Here's how the part is built. I have some questions about the finished solid (model axes, mm). Face numbers are marked on the shaded views. A direction names the side the tool comes from. Coordinates: 2 decimals unless noted, no trailing zeros.
```python
from build123d import *

# Parameters (mm, degrees)
SKETCH1_W                        = 15
SKETCH1_H                        = 6
MAIN_BODY_EXT_DEPTH              = 8.3
EMISSION_PATH_EXT_DEPTH          = 9
SKETCH3_R                        = 1.25
EMISSION_AND_GRIN_CUT_DEPTH      = 20.092931
SKETCH4_R                        = 1
DRUM_LENS_CUT_DEPTH              = 13
SKETCH41_R                       = 1
ADDTL_LIGHT_SOURCE_DEPTH         = 5
SKETCH5_W                        = 15
SKETCH5_H                        = 7.3
FILTERSET_CUT1_DEPTH             = 1
FILTERSET_CUT2_DEPTH             = 4
SKETCH10_R                       = 2.5
EMISSION_LENS_CUT_DEPTH          = 8.5
SKETCH15_R                       = 0.795
MAGNETS_CUT_DEPTH                = 0.9
SCREW_HOLES_CUT_DEPTH            = 20.507434
SCREW_HOLES_CUT_DEPTH_BACK       = 3
SKETCH18_R                       = 0.375
EXTERNAL_FILLET_1_R              = 1.5
CUT_EXTRUDE8_DEPTH               = 14.011149
CUT_EXTRUDE8_DEPTH_BACK          = 4
SKETCH28_R                       = 1.5
CUT_EXTRUDE9_DEPTH               = 3
CUT_EXTRUDE_ORIGINAL_LIGHT_DEPTH = 0.7
CUT_EXTRUDE_ADDTL_LIGHT_DEPTH    = 0.7
SKETCH29_R                       = 0.375
CUT_EXTRUDE11_DEPTH              = 2.5
SKETCH32_W                       = 2
SKETCH32_H                       = 2.36
CUT_EXTRUDE14_DEPTH              = 0.7
SKETCH45_W                       = 2.36
SKETCH45_H                       = 2
CUT_EXTRUDE19_DEPTH              = 0.7
CUT_EXTRUDE16_DEPTH              = 9
CUT_EXTRUDE17_REACH              = 13.945
SKETCH37_R                       = 2
BOSS_EXTRUDE2_DEPTH              = 1
SKETCH51_R                       = 0.356741
ADD_L_SCREW_HOLE_DEPTH           = 2


with BuildPart() as part:
    # Sketch1 → Main Body Ext (new body)
    with BuildSketch(Plane(origin=(0, 0, 0), x_dir=(1, 0, 0), z_dir=(0, 1, 0))):
        Rectangle(SKETCH1_W, SKETCH1_H)
    extrude(amount=MAIN_BODY_EXT_DEPTH)

    # Sketch8 → Emission Path Ext (add)
    with BuildSketch(Plane(origin=(0, 8.3, 0), x_dir=(1, 0, 0), z_dir=(0, 1, 0))):
        Polygon((-2.75, 3), (-1.5, 1.75), (-1.5, -3), (-7.5, -3), (-7.5, 3), align=None)
    extrude(amount=EMISSION_PATH_EXT_DEPTH)

    # Sketch3 → Emission and Grin Cut (cut, through all)
    with BuildSketch(Plane.XZ):
        with Locations(Location((-4.5, 0, 0), (0, 0, 270))):
            Circle(SKETCH3_R)
    extrude(amount=-EMISSION_AND_GRIN_CUT_DEPTH, mode=Mode.SUBTRACT)

    # Sketch4 → Drum Lens Cut (cut)
    with BuildSketch(Plane(origin=(7.5, 0, 0), x_dir=(0, 0, -1), z_dir=(1, 0, 0))):
        with Locations((0, 3)):
            Circle(SKETCH4_R)
    extrude(amount=-DRUM_LENS_CUT_DEPTH, mode=Mode.SUBTRACT)

    # Sketch41 → Addtl Light Source (cut)
    with BuildSketch(Plane(origin=(0, 8.3, 0), x_dir=(1, 0, 0), z_dir=(0, 1, 0))):
        with Locations(Location((1.5, 0, 0), (0, 0, 270))):
            Circle(SKETCH41_R)
    extrude(amount=-ADDTL_LIGHT_SOURCE_DEPTH, mode=Mode.SUBTRACT)

    # Sketch5 → FilterSet Cut1 (cut)
    with BuildSketch(Plane.XY.offset(3)):
        with Locations((0, 4.65)):
            Rectangle(SKETCH5_W, SKETCH5_H)
    extrude(amount=-FILTERSET_CUT1_DEPTH, mode=Mode.SUBTRACT)

    # Sketch6 → FilterSet Cut2 (cut)
    with BuildSketch(Plane.XY.offset(2)):
        with BuildLine():
            Line((5.3, 4.5), (5.3, 1.8))
            ThreePointArc((5.3, 1.8), (5.7, 1.4), (5.3, 1))
            Line((5.3, 1), (4.1, 1))
            ThreePointArc((4.1, 1), (3.7, 1.4), (4.1, 1.8))
            Line((4.1, 1.8), (4.1, 4.5))
            ThreePointArc((4.1, 4.5), (4.7, 5.1), (5.3, 4.5))
        make_face()
        with BuildLine():
            Line((-6.9, 7.9), (-6.9, 7.5))
            ThreePointArc((-6.9, 7.5), (-6.782843, 7.217157), (-6.5, 7.1))
            Line((-6.5, 7.1), (-2.5, 7.1))
            ThreePointArc((-2.5, 7.1), (-2.217157, 7.217157), (-2.1, 7.5))
            Line((-2.1, 7.5), (-2.1, 7.9))
            ThreePointArc((-2.1, 7.9), (-2.217157, 8.182843), (-2.5, 8.3))
            Line((-2.5, 8.3), (-6.5, 8.3))
            ThreePointArc((-6.5, 8.3), (-6.782843, 8.182843), (-6.9, 7.9))
        make_face()
        with BuildLine():
            Line((-2.605887, 6.591169), (-6.848528, 2.348528))
            ThreePointArc((-6.848528, 2.348528), (-6.848528, 1.5), (-6, 1.5))
            Line((-6, 1.5), (-1.757359, 5.742641))
            ThreePointArc((-1.757359, 5.742641), (-1.757359, 6.591169), (-2.605887, 6.591169))
        make_face()
        with BuildLine():
            Line((3.112092, 6.591169), (-1.130548, 2.348528))
            ThreePointArc((-1.130548, 2.348528), (-1.130548, 1.5), (-0.28202, 1.5))
            Line((-0.28202, 1.5), (3.96062, 5.742641))
            ThreePointArc((3.96062, 5.742641), (3.96062, 6.591169), (3.112092, 6.591169))
        make_face()
    extrude(amount=-FILTERSET_CUT2_DEPTH, mode=Mode.SUBTRACT)

    # Sketch10 → Emission Lens Cut (cut)
    with BuildSketch(Plane(origin=(0, 17.3, 0), x_dir=(1, 0, 0), z_dir=(0, 1, 0))):
        with Locations(Location((-4.5, 0, 0), (0, 0, 270))):
            Circle(SKETCH10_R)
    extrude(amount=-EMISSION_LENS_CUT_DEPTH, mode=Mode.SUBTRACT)

    # Sketch15 → Magnets Cut (cut)
    with BuildSketch(Plane.XZ):
        with Locations(Location((-6.25, -1.875, 0), (0, 0, 270))):
            Circle(SKETCH15_R)
        with Locations(Location((-6.25, 1.875, 0), (0, 0, 270))):
            Circle(SKETCH15_R)
        with Locations(Location((2.5, 0, 0), (0, 0, 270))):
            Circle(SKETCH15_R)
    extrude(amount=-MAGNETS_CUT_DEPTH, mode=Mode.SUBTRACT)

    # Sketch18 → Screw Holes Cut (cut, two sides: drawn at the far end of the back side and taken through both)
    with BuildSketch(Plane.XY.offset(2).offset(-SCREW_HOLES_CUT_DEPTH_BACK)):
        with Locations(Location((-6.5, 4, 0), (0, 0, 180))):
            Circle(SKETCH18_R)
        with Locations(Location((6, 5, 0), (0, 0, 180))):
            Circle(SKETCH18_R)
        with Locations((0.25, 1)):
            Circle(SKETCH18_R)
    extrude(amount=SCREW_HOLES_CUT_DEPTH + SCREW_HOLES_CUT_DEPTH_BACK, mode=Mode.SUBTRACT)

    # External Fillet 1
    # the kernel refuses this fillet: 1.5 mm, written as the material it takes off along each edge
    with BuildSketch(Plane(origin=(-7.5, -3.75, -3), x_dir=(1, 0, 0), z_dir=(0, 1, 0))) as external_fillet_1_piece_1:
        with BuildLine():
            CenterArc((EXTERNAL_FILLET_1_R, -EXTERNAL_FILLET_1_R), EXTERNAL_FILLET_1_R, 90, 90)
            Line((0, -EXTERNAL_FILLET_1_R), (0, 0))
            Line((0, 0), (EXTERNAL_FILLET_1_R, 0))
        make_face()
    extrude(amount=24.8, mode=Mode.SUBTRACT)
    with BuildSketch(Plane(origin=(-1.5, 8.3, 3), x_dir=(0, 0, -1), z_dir=(0, 1, 0))) as external_fillet_1_piece_2:
        with BuildLine():
            CenterArc((EXTERNAL_FILLET_1_R, EXTERNAL_FILLET_1_R), EXTERNAL_FILLET_1_R, 180, 90)
            Line((0, EXTERNAL_FILLET_1_R), (0, 0))
            Line((0, 0), (EXTERNAL_FILLET_1_R, 0))
        make_face()
    extrude(amount=12.75, mode=Mode.SUBTRACT)

    # Sketch28 → Cut-Extrude8 (cut, two sides: drawn at the far end of the back side and taken through both)
    with BuildSketch(Plane(origin=(0, 7.1, 0), x_dir=(1, 0, 0), z_dir=(0, 1, 0)).offset(-CUT_EXTRUDE8_DEPTH_BACK)):
        with Locations(Location((-4.5, 0, 0), (0, 0, 180))):
            Circle(SKETCH28_R)
    extrude(amount=CUT_EXTRUDE8_DEPTH + CUT_EXTRUDE8_DEPTH_BACK, mode=Mode.SUBTRACT)

    # Sketch14 → Cut-Extrude9 (cut)
    with BuildSketch(Plane.XZ):
        Polygon((7.5, -3), (7.5, -1.891585), (7.056634, -3), align=None)
    extrude(amount=-CUT_EXTRUDE9_DEPTH, mode=Mode.SUBTRACT)

    # Sketch12 → Cut-Extrude Original Light (cut)
    with BuildSketch(Plane(origin=(7.5, 0, 0), x_dir=(0, 0, -1), z_dir=(1, 0, 0))):
        with BuildLine():
            Line((1.6, 5.94), (-1.6, 5.94))
            Line((-1.6, 5.94), (-2, 5.94))
            Line((-2, 5.94), (-2, 1.33))
            Line((-2, 1.33), (1.6, 1.33))
            ThreePointArc((1.6, 1.33), (1.882843, 1.447157), (2, 1.73))
            Line((2, 1.73), (2, 5.54))
            ThreePointArc((2, 5.54), (1.882843, 5.822843), (1.6, 5.94))
        make_face()
    extrude(amount=-CUT_EXTRUDE_ORIGINAL_LIGHT_DEPTH, mode=Mode.SUBTRACT)

    # Sketch44 → Cut-Extrude Addtl Light (cut)
    with BuildSketch(Plane(origin=(0, 8.3, 0), x_dir=(1, 0, 0), z_dir=(0, 1, 0))):
        with BuildLine():
            Line((-0.17, -2), (4.44, -2))
            Line((4.44, -2), (4.44, 1.6))
            ThreePointArc((4.44, 1.6), (4.322843, 1.882843), (4.04, 2))
            Line((4.04, 2), (0.23, 2))
            ThreePointArc((0.23, 2), (-0.052843, 1.882843), (-0.17, 1.6))
            Line((-0.17, 1.6), (-0.17, -2))
        make_face()
    extrude(amount=-CUT_EXTRUDE_ADDTL_LIGHT_DEPTH, mode=Mode.SUBTRACT)

    # Sketch29 → Cut-Extrude11 (cut)
    with BuildSketch(Plane(origin=(7.5, 0, 0), x_dir=(0, 0, -1), z_dir=(1, 0, 0))):
        with Locations((2, 6.5)):
            Circle(SKETCH29_R)
    extrude(amount=-CUT_EXTRUDE11_DEPTH, mode=Mode.SUBTRACT)

    # Sketch32 → Cut-Extrude14 (cut)
    with BuildSketch(Plane(origin=(7.5, 0, 0), x_dir=(0, 0, -1), z_dir=(1, 0, 0))):
        with Locations((0, 7.12)):
            Rectangle(SKETCH32_W, SKETCH32_H)
    extrude(amount=-CUT_EXTRUDE14_DEPTH, mode=Mode.SUBTRACT)

    # Sketch45 → Cut-Extrude19 (cut)
    with BuildSketch(Plane(origin=(0, 8.3, 0), x_dir=(1, 0, 0), z_dir=(0, 1, 0))):
        with Locations((5.62, 0)):
            Rectangle(SKETCH45_W, SKETCH45_H)
    extrude(amount=-CUT_EXTRUDE19_DEPTH, mode=Mode.SUBTRACT)

    # Sketch33 → Cut-Revolve1 (revolve, cut)
    with BuildSketch(Plane.XY, mode=Mode.PRIVATE) as cut_revolve1_sk:
        with BuildLine():
            Line((6.8, 3), (5.3, 3))
            ThreePointArc((5.3, 3), (5.73934, 4.06066), (6.8, 4.5))
            Line((6.8, 4.5), (6.8, 3))
        make_face()
    revolve(cut_revolve1_sk.sketch.rotate(Axis((6.8, 3, 0), (-1, 0, 0)), 84.26086), axis=Axis((6.8, 3, 0), (-1, 0, 0)), mode=Mode.SUBTRACT)

    # Sketch47 → Cut-Revolve2 (revolve, cut)
    with BuildSketch(Plane(origin=(1.5, 0, 0), x_dir=(0, 0, -1), z_dir=(1, 0, 0))):
        with BuildLine():
            Line((-1.5, 7.6), (0, 7.6))
            Line((0, 7.6), (0, 6.137287))
            ThreePointArc((0, 6.137287), (-1.04756, 6.563498), (-1.5, 7.6))
        make_face()
    revolve(axis=Axis((1.5, 7.6, 0), (0, -1, 0)), mode=Mode.SUBTRACT)

    # Sketch36 → Cut-Extrude16 (cut)
    with BuildSketch(Plane(origin=(0, 17.3, 0), x_dir=(1, 0, 0), z_dir=(0, 1, 0))):
        with BuildLine():
            Line((-7.5, -1.5), (-7.5, -3))
            Line((-7.5, -3), (-6, -3))
            ThreePointArc((-6, -3), (-7.06066, -2.56066), (-7.5, -1.5))
        make_face()
    extrude(amount=-CUT_EXTRUDE16_DEPTH, mode=Mode.SUBTRACT)

    # Sketch37 → Cut-Extrude17 (cut, up to next)
    with BuildSketch(Plane(origin=(0, 8.8, 0), x_dir=(1, 0, 0), z_dir=(0, 1, 0)), mode=Mode.PRIVATE) as cut_extrude17_sk1:
        with Locations(Location((-4.5, 0, 0), (0, 0, 180))):
            Circle(SKETCH37_R)
    cut_extrude17_tool1 = extrude(cut_extrude17_sk1.sketch, amount=-CUT_EXTRUDE17_REACH, mode=Mode.PRIVATE) & part.part
    add(cut_extrude17_tool1.solids().sort_by_distance((-4.5, 8.8, 0))[0], mode=Mode.SUBTRACT)

    # Sketch49 → Boss-Extrude2 (add)
    with BuildSketch(Plane.XY.offset(2)):
        Polygon((7.5, 5.94), (7.5, 8.3), (4.448399, 8.3), (4.448399, 5.94), (7.025856, 5.94), (7.026388, 5.94), align=None)
    extrude(amount=BOSS_EXTRUDE2_DEPTH)

    # Sketch51 → Add'l Screw Hole (cut)
    with BuildSketch(Plane(origin=(0, 8.3, 0), x_dir=(1, 0, 0), z_dir=(0, 1, 0))):
        with Locations(Location((5, -2, 0), (0, 0, 270))):
            Circle(SKETCH51_R)
    extrude(amount=-ADD_L_SCREW_HOLE_DEPTH, mode=Mode.SUBTRACT)


solid = part.part
```
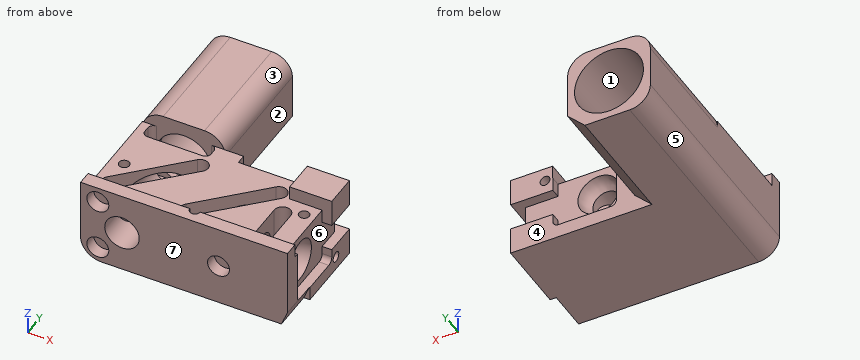
1. We'd pull the mould along Y, two halves only. Please class the marked faces 4, 5, 6 and 7: +Y half, -Y half, draft (parallel to the pull), parting line (faces both ways), or undercut.
2. On a 3-axis mill with a long thin cutter (end or side, diameter ignored), from which of +Z, -Z, +X, -X, +Y, -Y can I reach the whole of each face in a straight line? I mean the marked faces 1, 2 and 3. Say none if no direction works.
3. I need wall thicknesses on line 1 along X through (y, z) = (5.15, 0); line 2 along Y through (x, z) = (6.75, -0.1); line 3 along Y through (x, z) = (6.25, 1.15). Which ranges of each line are inside material? Lowest first, please.
4. For pin 1 (1.5 mm diameter, centred on y = 14, z = -2, fed in from +X); pin 2 (1.8 mm diameter, centred on y = 3, z = 0, fed in from +X), each with a flat end and sliding along its axis, tell me the tip position at first contact or that it passes through.
Response values:
1. face 4: +Y half
1. face 5: draft
1. face 6: undercut
1. face 7: -Y half
2. face 1: +Y
2. face 2: +Z, -Z, +X, +Y
2. face 3: +Z, +X, +Y
3. line 1: x = -7.5 to -6, -2.35 to 0.5, 3.37 to 5.66, 6.34 to 6.8
3. line 2: y = 0 to 1.5, 4.5 to 7.6
3. line 3: y = 0 to 2.21, 3.79 to 4.72, 5.28 to 8.3
4. pin 1: stops at x = -1.5
4. pin 2: stops at x = -5.77
